Answer from the drawing. Dimensions are ordinates in mm from the lowest x, y and z of the part. A direction names the side the tool comes from. Coordinates: 2 decimals unless noted, no trailing zeros. Write each loop counter-clockwise with the first axis right and the second up, starting at its lowest first coordinate (ties: lowest second). Pieces come first, ordered by that corner, then holes.
(1) Which of the six approach directions +Z, -Z, +X, -X, +Y, -Y give full straight-line access (tool end or side, diameter ignored) to the marked faces 1 and 2?
(2) Determine the mould class of the marked faces 3, 4 and 5 for opening direction X: pulls with the +X half, pulls with the -X half, needs draft (parallel to the pull), parting line crosses it, or undercut.
(3) The part is cut by section D-D, the plane z = 100. Determine the outline of the cut face in (x, y), and give its area (3 significant figures).
(4) Straight lines are drawn through the part: line 1 along Z through (x, y) = (130, 92); line 2 along Y through (x, z) = (74, 104); line 3 along Y through (x, z) = (74, 113). For each, find the intervals that lie inside material, in ascending order.
(5) The part is cut by section C-C, the plane y = 16.5. Determine the outline of the cut face in (x, z).
(6) Given pin 1 (5 mm diameter, centred on x = 68.5, z = 93.5, fed in from -Y); pin 2 (1.5 mm diameter, centred on x = 45.5, z = 28.5, fed in from -Y); pin 3 (4 mm diameter, centred on y = 47.5, z = 96, fed in from +X), each flat-ended and moving along its own axis, determine where each tip first touches the part or whether it passes through.
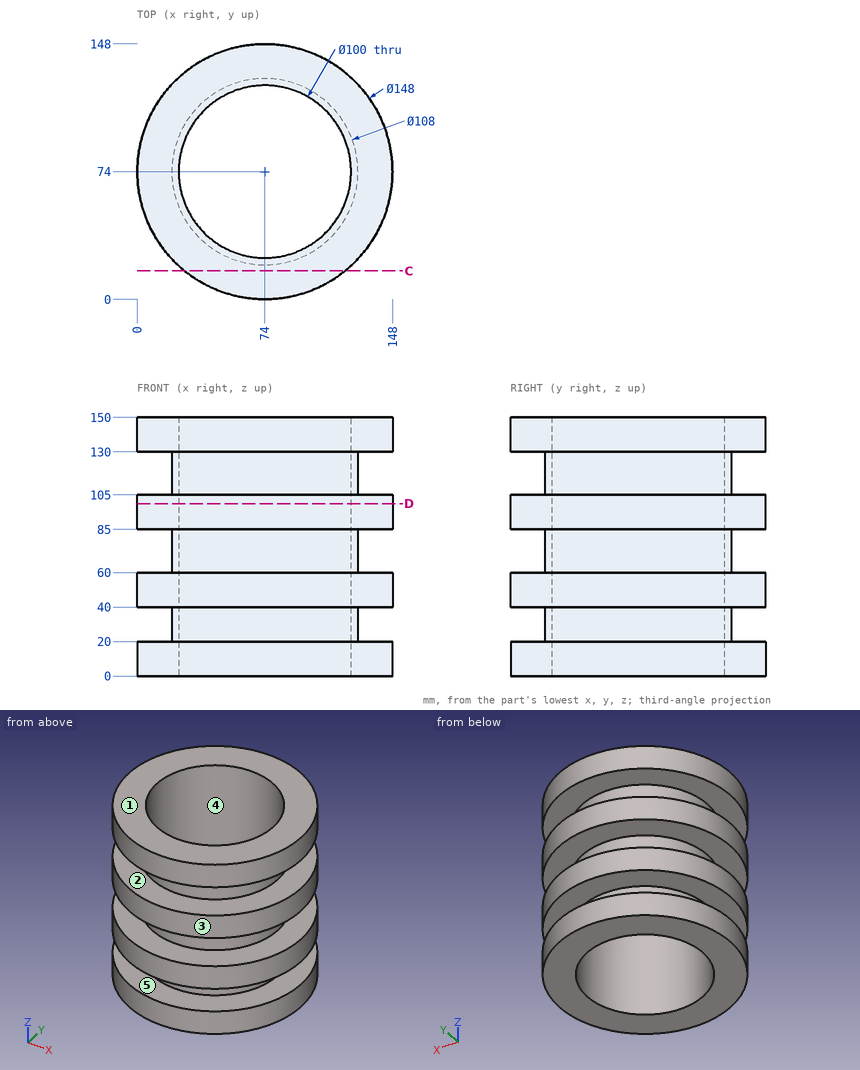
Computed:
1. face 1: +Z, +X, -X, +Y, -Y
1. face 2: none
2. face 3: parting line crosses it
2. face 4: undercut
2. face 5: needs draft
3. outline: circle Ø148 at (74, 74); hole circle Ø100 at (74, 74)
3. area: 9,350 mm2
4. line 1: z = 0 to 20, 40 to 60, 85 to 105, 130 to 150
4. line 2: y = 0 to 24, 124 to 148
4. line 3: y = 20 to 24, 124 to 128
5. outline: (27.42, 0) - (120.58, 0) - (120.58, 20) - (27.42, 20) - close; (27.42, 40) - (120.58, 40) - (120.58, 60) - (27.42, 60) - close; (27.42, 85) - (120.58, 85) - (120.58, 105) - (27.42, 105) - close; (27.42, 130) - (120.58, 130) - (120.58, 150) - (27.42, 150) - close
6. pin 1: stops at y = 0.06
6. pin 2: stops at y = 27.68
6. pin 3: stops at x = 143.83
